Read the model definition and answer for the solid it produces. Units are mm, in the model's axes. Give positions to 0.01 mm unless a question says otherwise; leave off trailing zeros. Write each loop counter-clockwise with the first axis right and the second up, starting at its lowest first coordinate (ties: lowest second). Pieces come first, ordered by that corner, then holes. Notation, with made-up numbers: M 2.5,75 L 13.5,75 A20 ccw 13.5,114 Z; hole C 37,82.25 d6. An arc over 180 degrees is marked long. Use a Markdown table: item, result. Add a question column.
Item 1: A cutting plane is placed at A-A on z = 12.5. Determine the outline of the cut face in (x, y), then the cut area to 3 significant figures.
Item 2: A cutting plane is placed at C-C on y = -23.25. Determine the outline of the cut face in (x, z).
Item 3: Consider probe 1 along X at (y, z) = (-11.5, 15.5); probe 2 along X at (y, z) = (-2.5, 6.5); probe 3 along Z at (x, y) = (-5, -13.5). Determine where each line is inside the solid, lowest interval first. Write a range as [from, to].
Item 4: Given P1, Ø5, axis at y = -23, z = -9, coming from the +X side; P2, Ø3, axis at x = 14, z = 14.5, coming from the +Y side, each flat-ended and moving along its own axis, determine where each tip first touches the part or whether it passes through.
Item 5: The mould has two halves that part along Z. Classify faces 1 (the flat face through (-29.03, -22.896, 2.261)), 2 (the cylindrical face through (-20.18, -12.88, 3.87)), 3 (the flat face through (-28.13, -22.26, -18.95)), 4 (the flat face through (-29.03, -12.52, 19.99)): pulls with the +Z half, pulls with the -Z half, needs draft (parallel to the pull), parting line crosses it, or undercut.
Item 6: A cutting plane is placed at B-B on x = -16.5. Determine the outline of the cut face in (y, z), then the cut area to 3 significant figures.
Item 7: A cutting plane is placed at D-D on z = -16. Determine the outline of the cut face in (x, y), then the cut area to 3 significant figures.
from build123d import *

# Parameters (mm, degrees)
F0_W     = 63.210748136
F0_H     = 44.9878275394
F1_DEPTH = 25.4
F3_D     = 25.4
F4_SIZE  = 5.08


with BuildPart() as f1:
    # F0 (on Front) → F1 (new body)
    with BuildSketch(Plane.XZ):
        Rectangle(F0_W, F0_H)
    extrude(amount=F1_DEPTH)

    # F3 (through all)
    with Locations(Plane(origin=(0, 0, 0), x_dir=(1, 0, 0), z_dir=(0, 1, 0))):
        with Locations((-8.0674383789, -7.687793579)):
            Hole(F3_D / 2)

    # F4
    f4_edges = [f1.edges().sort_by_distance(p)[0] for p in [
        (31.605374, -12.7, -22.493914),
        (31.605374, -12.7, 22.493914),
        (31.605374, 0, 0),
        (31.605374, -25.4, 0),
        (-31.605374, -12.7, 22.493914),
        (-31.605374, -12.7, -22.493914),
        (-31.605374, 0, 0),
        (-31.605374, -25.4, 0),
        (0, 0, -22.493914),
        (0, -25.4, -22.493914),
    ]]
    chamfer(f4_edges, length=F4_SIZE)


solid = f1.part
Filled in:
| question | item | result |
|---|---|---|
| 1 | outline | M -31.61,-20.32 L -26.53,-25.4 L -19.82,-25.4 L -19.82,0 L -26.53,0 L -31.61,-5.08 Z; M 3.69,-25.4 L 26.53,-25.4 L 31.61,-20.32 L 31.61,-5.08 L 26.53,0 L 3.69,0 Z |
| 1 | area | 957 mm² |
| 2 | outline | M -28.68,-17.41 L -26.53,-19.56 L 26.53,-19.56 L 28.68,-17.41 L 28.68,20.34 L 26.53,22.49 L -26.53,22.49 L -28.68,20.34 Z; hole C -8.07,7.69 d25.4 |
| 3 | probe 1 | [-31.61, -18.08], [1.95, 31.61] |
| 3 | probe 2 | [-29.03, -20.71], [4.58, 29.03] |
| 3 | probe 3 | [-22.49, -4.64], [20.01, 22.49] |
| 4 | P1 | x = 31.43 |
| 4 | P2 | y = 0 |
| 5 | face 1 | needs draft |
| 5 | face 2 | undercut |
| 5 | face 3 | pulls with the -Z half |
| 5 | face 4 | pulls with the +Z half |
| 6 | outline | M -25.4,-17.41 L -20.32,-22.49 L -5.08,-22.49 L 0,-17.41 L 0,-1.81 L -25.4,-1.81 Z; M -25.4,17.18 L 0,17.18 L 0,22.49 L -25.4,22.49 Z |
| 6 | area | 634 mm² |
| 7 | outline | M -31.61,-20.32 L -26.53,-25.4 L 26.53,-25.4 L 31.61,-20.32 L 31.61,-5.08 L 26.53,0 L -26.53,0 L -31.61,-5.08 Z |
| 7 | area | 1,550 mm² |
